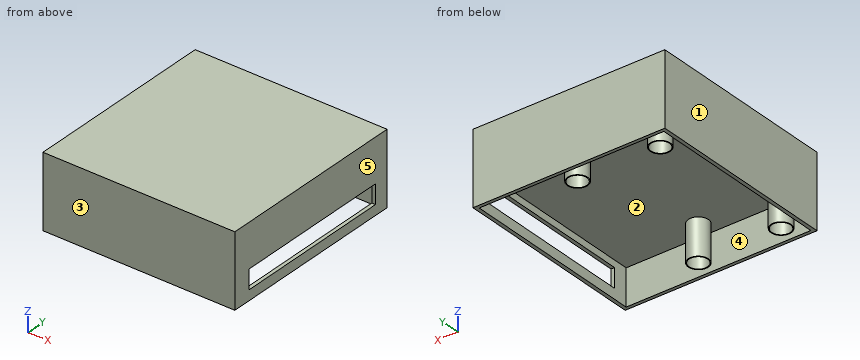
```python
from build123d import *

# Parameters (mm, degrees)
F0_W     = 29
F0_H     = 29.32
F0_W_2   = 27.91
F0_H_2   = 28.32
F0_R     = 1.525
F0_R_2   = 1.4
F1_DEPTH = 11
F2_DEPTH = 5.5
F3_W     = 24.3599908426
F3_H     = 2.9126071604
F4_DEPTH = 10


with BuildPart() as f1:
    # F0 (on Top) → F1 (new body)
    with BuildSketch(Plane.XY):
        with Locations((2, 1.5)):
            Rectangle(F0_W, F0_H)
        with Locations((2, 1.5)):
            Rectangle(F0_W_2, F0_H_2, mode=Mode.SUBTRACT)
        with Locations((2, 1.5)):
            Rectangle(F0_W_2, F0_H_2)
        with Locations((-9.435, -10.14)):
            Circle(F0_R, mode=Mode.SUBTRACT)
        with Locations((3.065, -10.14)):
            Circle(F0_R, mode=Mode.SUBTRACT)
        with Locations((-9.435, 13.14)):
            Circle(F0_R, mode=Mode.SUBTRACT)
        with Locations((3.065, 13.14)):
            Circle(F0_R, mode=Mode.SUBTRACT)
        with Locations((3.065, 13.14)):
            Circle(F0_R)
        with Locations((3.065, 13.14)):
            Circle(F0_R_2, mode=Mode.SUBTRACT)
        with Locations((3.065, -10.14)):
            Circle(F0_R)
        with Locations((3.065, -10.14)):
            Circle(F0_R_2, mode=Mode.SUBTRACT)
        with Locations((-9.435, -10.14)):
            Circle(F0_R)
        with Locations((-9.435, -10.14)):
            Circle(F0_R_2, mode=Mode.SUBTRACT)
        with Locations((-9.435, 13.14)):
            Circle(F0_R)
        with Locations((-9.435, 13.14)):
            Circle(F0_R_2, mode=Mode.SUBTRACT)
        with Locations((3.065, 13.14)):
            Circle(F0_R_2)
        with Locations((3.065, -10.14)):
            Circle(F0_R_2)
        with Locations((-9.435, -10.14)):
            Circle(F0_R_2)
        with Locations((-9.435, 13.14)):
            Circle(F0_R_2)
    extrude(amount=F1_DEPTH)

    # F0 (on Top) → F2 (cut)
    with BuildSketch(Plane.XY):
        with Locations((2, 1.5)):
            Rectangle(F0_W_2, F0_H_2)
        with Locations((-9.435, -10.14)):
            Circle(F0_R, mode=Mode.SUBTRACT)
        with Locations((3.065, -10.14)):
            Circle(F0_R, mode=Mode.SUBTRACT)
        with Locations((-9.435, 13.14)):
            Circle(F0_R, mode=Mode.SUBTRACT)
        with Locations((3.065, 13.14)):
            Circle(F0_R, mode=Mode.SUBTRACT)
        with Locations((-9.435, -10.14)):
            Circle(F0_R_2)
        with Locations((3.065, -10.14)):
            Circle(F0_R_2)
        with Locations((3.065, 13.14)):
            Circle(F0_R_2)
        with Locations((-9.435, 13.14)):
            Circle(F0_R_2)
    extrude(amount=F2_DEPTH, mode=Mode.SUBTRACT)

    # F3 (on face) → F4 (cut)
    with BuildSketch(Plane.YZ.offset(16.5)):
        with Locations((1.7549390905, 2.9909135192)):
            Rectangle(F3_W, F3_H)
    extrude(amount=-F4_DEPTH, mode=Mode.SUBTRACT)


solid = f1.part
```
Design review of the part built by this model. Coordinates are the model's own, in mm. Face numbers are marked on the shaded views. A direction names the side the tool comes from. Round coordinates to 2 decimals unless told otherwise and drop trailing zeros. Order: outer loops, then holes, each group sorted by start corner. A loop starts at its lowest first (then second) coordinate and runs counter-clockwise, first axis right, second up. Notation, with made-up numbers: M 44.5,-4.5 L 73.5,-4.5 A14 cw 73.5,18.5 Z; hole C -36,5 d8. An arc over 180 degrees is marked long. Put each result on its own line as item: value.
Q1. Consider section A-A (z = 2.5). State how many separate pieces and enclosed holes the cut face has, and give its area (3 significant figures).
Reported:
separate pieces: 5
enclosed holes: 4
area: 51.2 mm²
Q2. Machinability: for the marked faces 4 and 5, which of the approach directions +Z, -Z, +X, -X, +Y, -Y give a long, thin tool a straight path to every point of the face, cutting with its end or side? Answer none if there is none.
Reported:
face 4: -Z
face 5: +Z, -Z, +X, +Y, -Y
Q3. Consider section C-C (x = -6). State the section outline as (y, z) points, and give its area (3 significant figures).
Reported:
outline: M -13.16,0 L -12.66,0 L -12.66,5.5 L 15.66,5.5 L 15.66,0 L 16.16,0 L 16.16,11 L -13.16,11 Z
area: 167 mm²
Q4. Consider section D-D (y = 13.14). State the section outline as (x, z) points (3 decimals), and give its area (3 significant figures).
Reported:
outline: M -12.5,0 L -11.955,0 L -11.955,5.5 L -10.96,5.5 L -10.96,0 L -10.835,0 L -10.835,5.5 L -8.035,5.5 L -8.035,0 L -7.91,0 L -7.91,5.5 L 1.54,5.5 L 1.54,0 L 1.665,0 L 1.665,5.5 L 4.465,5.5 L 4.465,0 L 4.59,0 L 4.59,5.5 L 15.955,5.5 L 15.955,4.447 L 16.5,4.447 L 16.5,11 L -12.5,11 Z; M 15.955,0 L 16.5,0 L 16.5,1.535 L 15.955,1.535 Z
area: 167 mm²
Q5. To check wall thickness, follow line 1 (Y direction, x = 0.5, z = 1); line 2 (X direction, y = 6.75, z = 1) (3 decimals); line 3 (Z direction, x = -7.25, y = 5.25). State the ranges of each line that lie inside material, in increasing order.
Reported:
line 1: -13.16 to -12.66, 15.66 to 16.16
line 2: -12.5 to -11.955, 15.955 to 16.5
line 3: 5.5 to 11
Q6. Consider section B-B (y = 9). State the section outline as (x, z) points (3 decimals), and give its area (3 significant figures).
Reported:
outline: M -12.5,0 L -11.955,0 L -11.955,5.5 L 15.955,5.5 L 15.955,4.447 L 16.5,4.447 L 16.5,11 L -12.5,11 Z; M 15.955,0 L 16.5,0 L 16.5,1.535 L 15.955,1.535 Z
area: 164 mm²
Q7. Insertion check: pin 1 Ø3 at (y, z) = (-3, 4) entering from +X; pin 2 Ø2 at (x, y) = (3.065, -10.14) entering from -Z. Each pin has a flat end and moves straight along its axis. Give the tip position at first contact, or say it passes through.
Reported:
pin 1: x = 16.5
pin 2: z = 5.5
Q8. Draft analysis for pull direction X (two halves, no side actions). For the marked faces 1, 2 and 3, state which applies: released by +X, released by -X, zero draft, split by the parting line, or undercut.
Reported:
face 1: released by -X
face 2: undercut
face 3: zero draft
